Here's how the part is built. I have some questions about the finished solid (model axes, mm). A direction names the side the tool comes from. Round coordinates to 2 decimals unless told otherwise and drop trailing zeros. Order: outer loops, then holes, each group sorted by start corner. A loop starts at its lowest first (then second) coordinate and runs counter-clockwise, first axis right, second up.
```python
from build123d import *

# Parameters (mm, degrees)
F1_DEPTH = 12.5
F3_DEPTH = 12.5


with BuildPart() as f1:
    # F0 (on Right) → F1 (new body, symmetric)
    with BuildSketch(Plane.YZ):
        with BuildLine():
            Line((0, -17), (0, -12))
            ThreePointArc((0, -12), (-9.8315408875, -6.8804653751), (-11.2742627767, 4.1098660371))
            Line((-11.2742627767, 4.1098660371), (-12.6953165638, 5.5172061289))
            ThreePointArc((-12.6953165638, 5.5172061289), (-12.9247401764, -9.4495895167), (0, -17))
        make_face()
        with BuildLine():
            ThreePointArc((11.2742627767, 4.1098660371), (11.8171729555, 2.0867255066), (12, 0))
            ThreePointArc((12, 0), (8.4852813742, -8.4852813742), (0, -12))
            Line((0, -12), (0, -17))
            ThreePointArc((0, -17), (12.9247401764, -9.4495895167), (12.6953165638, 5.5172061289))
            Line((12.6953165638, 5.5172061289), (11.2742627767, 4.1098660371))
        make_face()
    extrude(amount=F1_DEPTH, both=True)

    # F2 (on Front) → F3 (join, symmetric)
    with BuildSketch(Plane.XZ):
        with BuildLine():
            ThreePointArc((0, -18.6252225989), (6.0382661769, -20.3380196492), (10.2778672238, -24.9662066724))
            Line((10.2778672238, -24.9662066724), (12.4753578975, -24.9662066724))
            ThreePointArc((12.4753578975, -24.9662066724), (7.944802109, -17.8816045994), (0, -15.1252225989))
            Line((0, -15.1252225989), (0, -18.6252225989))
        make_face()
        with BuildLine():
            Line((-12.4753578975, -24.9662066724), (-10.2778672238, -24.9662066724))
            ThreePointArc((-10.2778672238, -24.9662066724), (-6.0382661769, -20.3380196492), (0, -18.6252225989))
            Line((0, -18.6252225989), (0, -15.1252225989))
            ThreePointArc((0, -15.1252225989), (-7.944802109, -17.8816045994), (-12.4753578975, -24.9662066724))
        make_face()
    extrude(amount=F3_DEPTH, both=True)


solid = f1.part
```
1. If we section it at D-D, the plane x = 6.25: Write out the boundary of the cut face in (y, z).
Evaluation:
outline: (-12.7, 5.52) arc R14.84 ccw to (-2.71, -16.75) - (-12.5, -16.75) - (-12.5, -20.47) - (12.5, -20.47) - (12.5, -16.75) - (2.71, -16.75) arc R14.84 ccw to (12.7, 5.52) - (11.27, 4.11) arc R12 cw (long way) to (-11.27, 4.11) - close
2. I need wall thicknesses on probe 1 along Y at (x, z) = (7.5, -20); probe 2 along Z at (x, y) = (1.5, 10.75); probe 3 along Y at (x, z) = (5.75, 0). Which ranges of each line are inside material? Lowest first, please.
Evaluation:
probe 1: y = -12.5 to 12.5
probe 2: z = -18.72 to -15.21, -12.39 to -5.33
probe 3: y = -14.68 to -12, 12 to 14.68
3. I'm going to push flat-ended pins straight in: P1, Ø8, axis at x = -3, z = -21, coming from the -Y side; P2, Ø2, axis at x = -5, z = -9, coming from the +Y side; P3, Ø8, axis at x = -3, z = -19.5, coming from the +Y side. Where does each tip first touch, or does it pass through?
Evaluation:
P1: stops at y = -12.5
P2: stops at y = 13.64
P3: stops at y = 12.5
4. If we mould it in two halves opening along Y, with no side actions, what happens to faces 1 (the flat face through (-11, 0, -24.966)), 2 (the flat face through (0, -12.5, -18)), 3 (the flat face through (0.18, 11.99, 4.82))? For each: released by +Y, released by -Y, zero draft, split by the parting line, or undercut.
Evaluation:
face 1: zero draft
face 2: released by -Y
face 3: undercut
5. If we section it at C-C, the plane y = -3.5: Write out the boundary of the cut face in (x, z).
Evaluation:
outline: (-12.5, -16.58) - (-5.94, -16.58) arc R12.83 ccw to (-12.48, -24.97) - (-10.28, -24.97) arc R11.5 cw to (10.28, -24.97) - (12.48, -24.97) arc R12.83 ccw to (5.94, -16.58) - (12.5, -16.58) - (12.5, -11.48) - (-12.5, -11.48) - close
6. On a 3-axis mill with a long thin cutter (end or side, diameter ignored), from which of +Z, -Z, +X, -X, +Y, -Y can I reach the whole of each face in a straight line? I mean faces 4 (the flat face through (-12.5, 1, -12.4)), 5 (the cylindrical face through (-2.603, -7.108, -15.187)), 6 (the flat face through (0.18, -11.97, 4.8)), 7 (the flat face through (12.5, 1, -12.4)), 8 (the flat face through (0, 12.5, -18)). Say none if no direction works.
Evaluation:
face 4: +Z, -Z, -X, +Y, -Y
face 5: none
face 6: +Z, +X, -X
face 7: +Z, -Z, +X, +Y, -Y
face 8: -Z, +X, -X, +Y
7. If we section it at B-B, the plane z = -1: Write out the boundary of the cut face in (x, y), and give its area (3 significant figures).
Evaluation:
outline: (-12.5, -14.79) - (12.5, -14.79) - (12.5, -11.96) - (-12.5, -11.96) - close; (-12.5, 11.96) - (12.5, 11.96) - (12.5, 14.79) - (-12.5, 14.79) - close
area: 142 mm2
8. If we section it at A-A, the plane x = -8.5: Write out the boundary of the cut face in (y, z), and give its area (3 significant figures).
Evaluation:
outline: (-12.7, 5.52) arc R14.84 ccw (long way) to (12.7, 5.52) - (11.27, 4.11) arc R12 cw (long way) to (-11.27, 4.11) - close; (-12.5, -22.38) - (12.5, -22.38) - (12.5, -18.35) - (-12.5, -18.35) - close
area: 307 mm2
